Autodesk Fusion 360 part; units mm, degrees
sketch "Sketch1" plane through (0, 0, 0) normal (0, 1, 0) x (1, 0, 0)
  line L0 (0, 0) -> (80, 0)
  line L1 (80, 0) -> (80, 100)
  line L2 (80, 100) -> (0, 100)
  line L3 (0, 100) -> (0, 0)
  circle A0 centre (4, 96) radius 1.5
  circle A1 centre (76, 96) radius 1.5
  circle A2 centre (76, 4) radius 1.5
  circle A3 centre (4, 4) radius 1.5
  line L4 (40, 100) -> (40, 0) construction
  line L5 (0, 50) -> (80, 50) construction
  line L6 (4, 96) -> (40, 96) construction
  line L7 (76, 96) -> (76, 50) construction
  line L8 (76, 96) -> (40, 96) construction
  line L9 (76, 50) -> (76, 4) construction
  dimension "d1" = 80
  dimension "d2" = 100
  dimension "d3" = 3
  dimension "d4" = 72
  dimension "d5" = 92
extrude "Extrude1" add sketch "Sketch1" along normal blind 1.6
sketch "Sketch2" plane through (0, 1.6, 0) normal (0, 1, 0) x (-1, 0, 0)
  circle A0 centre (-4, -96) radius 1.5
  circle A1 centre (-4, -4) radius 1.5
  circle A2 centre (-76, -96) radius 1.5
  circle A3 centre (-76, -4) radius 1.5
  line L0 (0, -100) -> (0, 0)
  line L1 (0, 0) -> (-80, 0)
  line L2 (-80, 0) -> (-80, -100)
  line L3 (-80, -100) -> (0, -100)
  line L4 (-58, -89.6377) -> (-80, -89.6377)
  line L5 (-80, -89.6377) -> (-80, -73.1377)
  line L6 (-80, -73.1377) -> (-58, -73.1377)
  line L7 (-58, -73.1377) -> (-58, -89.6377)
  line L8 (-58, -69.1377) -> (-80, -69.1377)
  line L9 (-80, -69.1377) -> (-80, -52.6377)
  line L10 (-80, -52.6377) -> (-58, -52.6377)
  line L11 (-58, -52.6377) -> (-58, -69.1377)
  line L12 (-58, -48.6377) -> (-80, -48.6377)
  line L13 (-80, -48.6377) -> (-80, -32.1377)
  line L14 (-80, -32.1377) -> (-58, -32.1377)
  line L15 (-58, -32.1377) -> (-58, -48.6377)
  line L16 (-58, -28.1377) -> (-80, -28.1377)
  line L17 (-80, -28.1377) -> (-80, -11.6377)
  line L18 (-80, -11.6377) -> (-58, -11.6377)
  line L19 (-58, -11.6377) -> (-58, -28.1377)
  line L20 (0, -20) -> (-14.1052, -20)
  line L21 (-14.1052, -20) -> (-14.1052, -12.0995)
  line L22 (-14.1052, -12.0995) -> (0, -12.0995)
  line L23 (0, -12.0995) -> (0, -20)
  dimension "d8" = 16.5
  dimension "d9" = 22
  dimension "d10" = 4
  dimension "d11" = 4
  dimension "d12" = 4
extrude "Extrude2" add sketch "Sketch2" along normal blind 13.8 contours L2 L4 L5 L6 L7 | L2 L8 L9 L10 L11 | L2 L16 L17 L18 L19 | L2 L12 L13 L14 L15
extrude "Extrude3" add sketch "Sketch2" along normal blind 11 contours L0 L20 L21 L22 L23
sketch "Sketch3" plane through (0, 1.6, 0) normal (0, 1, 0) x (-1, 0, 0)
The model under review builds one solid part; all positions refer to its coordinate system, in mm. A direction names the side the tool comes from. Coordinates: 2 decimals unless noted, no trailing zeros. Write each loop counter-clockwise with the first axis right and the second up, starting at its lowest first coordinate (ties: lowest second). Pieces come first, ordered by that corner, then holes. Notation, with made-up numbers: (-38, -39.5) - (4, -39.5) arc R14 cw to (4, -26.5) - close; hole circle Ø2 at (-20.5, 30). An arc over 180 degrees is marked (long way). Answer as a JSON object with one key per item and string values. Group by question number.
1. Mouldability with a two-part tool opening along X and no side actions: class faces 4 (the face through (76.806, 0.789, -94.735)), 5 (the face through (80, 1, -49)), 6 (the face through (7, 7, -12.1)) as pulls with the +X half, pulls with the -X half, needs draft (parallel to the pull), parting line crosses it, or undercut.
2. Add section B-B (z = -96). Give the boundary of the cut face in (x, y).
3. Add section D-D (z = -61). Give the boundary of the cut face in (x, y).
4. Clearance check with flat-ended pins moving along their axes: pin 1 Ø4 at (x, y) = (65, 5.5) entering from -Z; pin 2 Ø5 at (x, z) = (4, -4) entering from +Y; pin 3 Ø8 at (y, z) = (6.5, -87) entering from -X. State where each tip first meets the part, or that it passes through.
5. Add section A-A (x = 4). Give the boundary of the cut face in (y, z), plus the area to 3 significant figures.
6. Machinability: for faces 1 (the face through (69, 8, -11.638)), 2 (the face through (69, 8, -52.638)), 3 (the face through (69, 8, -89.638)), which of the approach directions +Z, -Z, +X, -X, +Y, -Y give a long, thin tool a straight path to every point of the face, cutting with its end or side? Answer none if there is none.
7. To check wall thickness, follow probe 1 along X at (y, z) = (0.55, -4); probe 2 along Z at (x, y) = (70, 6); probe 3 along Z at (x, y) = (76, 1.1). State the ranges of each line that lie inside material, in increasing order.
8. Add section C-C (y = 7). Give the boundary of the cut face in (x, z), plus the area to 3 significant figures.
Findings:
{
 "1": {"face 4": "undercut", "face 5": "pulls with the +X half", "face 6": "needs draft"},
 "2": {"outline": "(0, 0) - (2.5, 0) - (2.5, 1.6) - (0, 1.6) - close; (5.5, 0) - (74.5, 0) - (74.5, 1.6) - (5.5, 1.6) - close; (77.5, 0) - (80, 0) - (80, 1.6) - (77.5, 1.6) - close"},
 "3": {"outline": "(0, 0) - (80, 0) - (80, 15.4) - (58, 15.4) - (58, 1.6) - (0, 1.6) - close"},
 "4": {"pin 1": "z = -89.64", "pin 2": "y = 1.6", "pin 3": "x = 58"},
 "5": {"outline": "(0, -100) - (1.6, -100) - (1.6, -97.5) - (0, -97.5) - close; (0, -94.5) - (1.6, -94.5) - (1.6, -20) - (12.6, -20) - (12.6, -12.1) - (1.6, -12.1) - (1.6, -5.5) - (0, -5.5) - close; (0, -2.5) - (1.6, -2.5) - (1.6, 0) - (0, 0) - close", "area": "237 mm²"},
 "6": {"face 1": "+Z, +X, -X, +Y", "face 2": "+X, -X, +Y", "face 3": "-Z, +X, -X, +Y"},
 "7": {"probe 1": "0 to 2.5, 5.5 to 74.5, 77.5 to 80", "probe 2": "-89.64 to -73.14, -69.14 to -52.64, -48.64 to -32.14, -28.14 to -11.64", "probe 3": "-100 to -97.5, -94.5 to -5.5, -2.5 to 0"},
 "8": {"outline": "(0, -20) - (14.11, -20) - (14.11, -12.1) - (0, -12.1) - close; (58, -89.64) - (80, -89.64) - (80, -73.14) - (58, -73.14) - close; (58, -69.14) - (80, -69.14) - (80, -52.64) - (58, -52.64) - close; (58, -48.64) - (80, -48.64) - (80, -32.14) - (58, -32.14) - close; (58, -28.14) - (80, -28.14) - (80, -11.64) - (58, -11.64) - close", "area": "1,560 mm²"}
}
